Input: part model. Units: mm. Frame: model coordinates. A direction names the side the tool comes from. Round coordinates to 2 decimals unless told otherwise and drop trailing zeros. Write each loop counter-clockwise with the first axis right and the second up, starting at its lowest first coordinate (ties: lowest second). Pieces come first, ordered by that corner, then holes. Notation, with made-up numbers: M 82.5,-35 L 115.5,-35 A18 cw 115.5,-6 Z; hole C -1,7.25 d9. An arc over 180 degrees is marked long. Write each question's results on one line, items separated by ' | '. Start each with the question number.
```python
from build123d import *

# Parameters (mm, degrees)
F1_DEPTH = 18
F2_R     = 3.25
F3_DEPTH = 3
F5_W     = 45
F5_H     = 17.2675769106
F6_DEPTH = 1
F7_R     = 1.75
F8_DEPTH = 25
F9_R     = 3
F10_R    = 1
F11_R    = 3
F12_R    = 1
F13_R    = 1
F14_R    = 1
F15_R    = 1
F16_R    = 1
F17_R    = 2
F18_R    = 1
F19_R    = 2
F20_R    = 1


with BuildPart() as f1:
    # F0 (on Top) → F1 (new body)
    with BuildSketch(Plane.XY):
        Polygon((22.5, 16), (-22.5, 16), (-22.5, -3), (-21.5, -3), (-21.5, 15), (21.5, 15), (21.5, -3), (22.5, -3), align=None)
    extrude(amount=F1_DEPTH)

    # F2 (on Top) → F3 (join)
    with BuildSketch(Plane.XY):
        with Locations((-21.5, -5.55)):
            Circle(F2_R)
        with Locations((21.5, -5.55)):
            Circle(F2_R)
    extrude(amount=F3_DEPTH)

    # F5 (on offset) → F6 (join)
    with BuildSketch(Plane.XY.offset(18)):
        with Locations((0, 7.3662115447)):
            Rectangle(F5_W, F5_H)
    extrude(amount=-F6_DEPTH)

    # F7 (on Top) → F8 (cut)
    with BuildSketch(Plane.XY):
        with Locations((21.5, -5.55)):
            Circle(F7_R)
        with Locations((-21.5, -5.55)):
            Circle(F7_R)
    extrude(amount=F8_DEPTH, mode=Mode.SUBTRACT)

    # F9
    f9_edges = [f1.edges().sort_by_distance(p)[0] for p in [
        (22.5, -2.457671, 1.5),
    ]]
    fillet(f9_edges, radius=F9_R)

    # F10
    f10_edges = [f1.edges().sort_by_distance(p)[0] for p in [
        (22.5, -2.728835, 3),
    ]]
    fillet(f10_edges, radius=F10_R)

    # F11
    f11_edges = [f1.edges().sort_by_distance(p)[0] for p in [
        (-22.5, -2.457671, 1.5),
    ]]
    fillet(f11_edges, radius=F11_R)

    # F12
    f12_edges = [f1.edges().sort_by_distance(p)[0] for p in [
        (-22.5, -2.728835, 3),
    ]]
    fillet(f12_edges, radius=F12_R)

    # F13
    f13_edges = [f1.edges().sort_by_distance(p)[0] for p in [
        (-22.5, 16, 9),
    ]]
    fillet(f13_edges, radius=F13_R)

    # F14
    f14_edges = [f1.edges().sort_by_distance(p)[0] for p in [
        (22.5, 16, 9),
    ]]
    fillet(f14_edges, radius=F14_R)

    # F15
    f15_edges = [f1.edges().sort_by_distance(p)[0] for p in [
        (-21.5, -1.267577, 17.5),
    ]]
    fillet(f15_edges, radius=F15_R)

    # F16
    f16_edges = [f1.edges().sort_by_distance(p)[0] for p in [
        (21.5, -1.267577, 17.5),
    ]]
    fillet(f16_edges, radius=F16_R)

    # F17
    f17_edges = [f1.edges().sort_by_distance(p)[0] for p in [
        (-21.5, -2.3, 1.5),
    ]]
    fillet(f17_edges, radius=F17_R)

    # F18
    f18_edges = [f1.edges().sort_by_distance(p)[0] for p in [
        (-21.5, -2.65, 3),
    ]]
    fillet(f18_edges, radius=F18_R)

    # F19
    f19_edges = [f1.edges().sort_by_distance(p)[0] for p in [
        (21.5, -2.3, 1.5),
    ]]
    fillet(f19_edges, radius=F19_R)

    # F20
    f20_edges = [f1.edges().sort_by_distance(p)[0] for p in [
        (21.5, -2.65, 3),
    ]]
    fillet(f20_edges, radius=F20_R)


solid = f1.part
```
1. Cut plane D-D on x = 16. Output: boundary loops of the cut face in (y, z).
2. Cut plane A-A on y = -5.55. Output: boundary loops of the cut face in (x, z).
3. Draft query along Y for faces 1 (the face through (-21.5, 6, 9)), 2 (the face through (21.215, -1.568, 17.493)), 3 (the face through (22.199, 15.715, 8.874)). Return one class per face: +Y half, -Y half, draft (parallel to the pull), parting line (faces both ways), or undercut.
4. Line query: L1, parallel to X at y = -5.55, z = 1.25; L2, parallel to X at y = 3, z = 15.75; L3, parallel to X at y = -7, z = 2. Output: solid intervals per line, ascending. Write a range as from..to.
5. Access query for faces 4 (the face through (-21.3, -2.1, 3.4)), 5 (the face through (-21.171, -1.795, 1.528)), 6 (the face through (-22, -3, 10)). Directions: +Z, -Z, +X, -X, +Y, -Y. A direction counts if a zero-diameter tool reaches every point of the face in a straight line with its end or side. Return the directions, or none.
6. Cut plane B-B on z = 15.5. Output: boundary loops of the cut face in (x, y).
7. Contact query for flat-ended pins moving along their axis: P1, Ø4, axis at x = 21.5, y = -5.55, coming from the +Z side; P2, Ø1.5, axis at x = -6, y = 1.5, coming from the -Z side; P3, Ø2.5, axis at x = 21.5, z = 14, coming from the -Y side. Output: stop coordinate, or through.
8. Cut plane C-C on y = 10.5. Output: boundary loops of the cut face in (x, z).
Answers follow:
1) outline: M -1.27,17 L 15,17 L 15,0 L 16,0 L 16,18 L -1.27,18 Z
2) outline: M -24.75,0 L -23.25,0 L -23.25,3 L -24.75,3 Z; M -19.75,0 L -18.25,0 L -18.25,3 L -19.75,3 Z; M 18.25,0 L 19.75,0 L 19.75,3 L 18.25,3 Z; M 23.25,0 L 24.75,0 L 24.75,3 L 23.25,3 Z
3) face 1: undercut | face 2: -Y half | face 3: +Y half
4) L1: x = -24.75..-23.25, -19.75..-18.25, 18.25..19.75, 23.25..24.75 | L2: x = -22.5..-21.5, 21.5..22.5 | L3: x = -24.41..-22.48, -20.52..-18.59, 18.59..20.52, 22.48..24.41
5) face 4: -Y | face 5: -Z | face 6: +Z, +X, -X, -Y
6) outline: M -22.5,-3 L -21.5,-3 L -21.5,15 L 21.5,15 L 21.5,-3 L 22.5,-3 L 22.5,15 A1 ccw 21.5,16 L -21.5,16 A1 ccw -22.5,15 Z
7) P1: stops at z = 3 | P2: stops at z = 17 | P3: stops at y = -3
8) outline: M -22.5,0 L -21.5,0 L -21.5,17 L 21.5,17 L 21.5,0 L 22.5,0 L 22.5,18 L -22.5,18 Z
